Study the drawing (mm; zero at the part's minimum x, y, z) and answer. Coordinates: 2 decimals unless noted, no trailing zeros. Write each loop counter-clockwise with the first axis right and the second up, starting at its lowest first coordinate (ties: lowest second). Pieces come first, ordered by that corner, then holes. Notation, with made-up numbers: (-36, 87.25) -> (-21, 87.25) arc R28 ccw to (-21, 106.25) -> close; hole circle Ø1 at (-19.75, 72). An arc over 180 degrees is marked (long way). Answer in a Markdown table with one row per item. Add a question column.
Item 1: Given pin 1 Ø4 at (x, y) = (17, 5) entering from -Z; pin 2 Ø1 at (y, z) = (4.5, 19.5) entering from +X; pin 3 Ø6 at (x, z) = (146.05, 6.35) entering from +Y, each flat-ended and moving along its own axis, determine where each tip first touches the part or whether it passes through.
Item 2: Section D-D on x = 123 is taken. Write down the section's boundary in (y, z), then the cut area to 3 significant figures.
Item 3: Section C-C on z = 90.5 is taken. Write down the section's boundary in (x, y), then the cut area to 3 significant figures.
Item 4: Section A-A on x = 6.35 is taken. Write down the section's boundary in (y, z), then the cut area to 3 significant figures.
Item 5: Straight lines are drawn through the part: line 1 (Z direction, x = 6.35, y = 1.85); line 2 (Z direction, x = 82, y = 3). For each, find the intervals that lie inside material, in ascending order. Write a range as from..to.
Item 6: Section B-B on z = 6.35 is taken. Write down the section's boundary in (x, y).
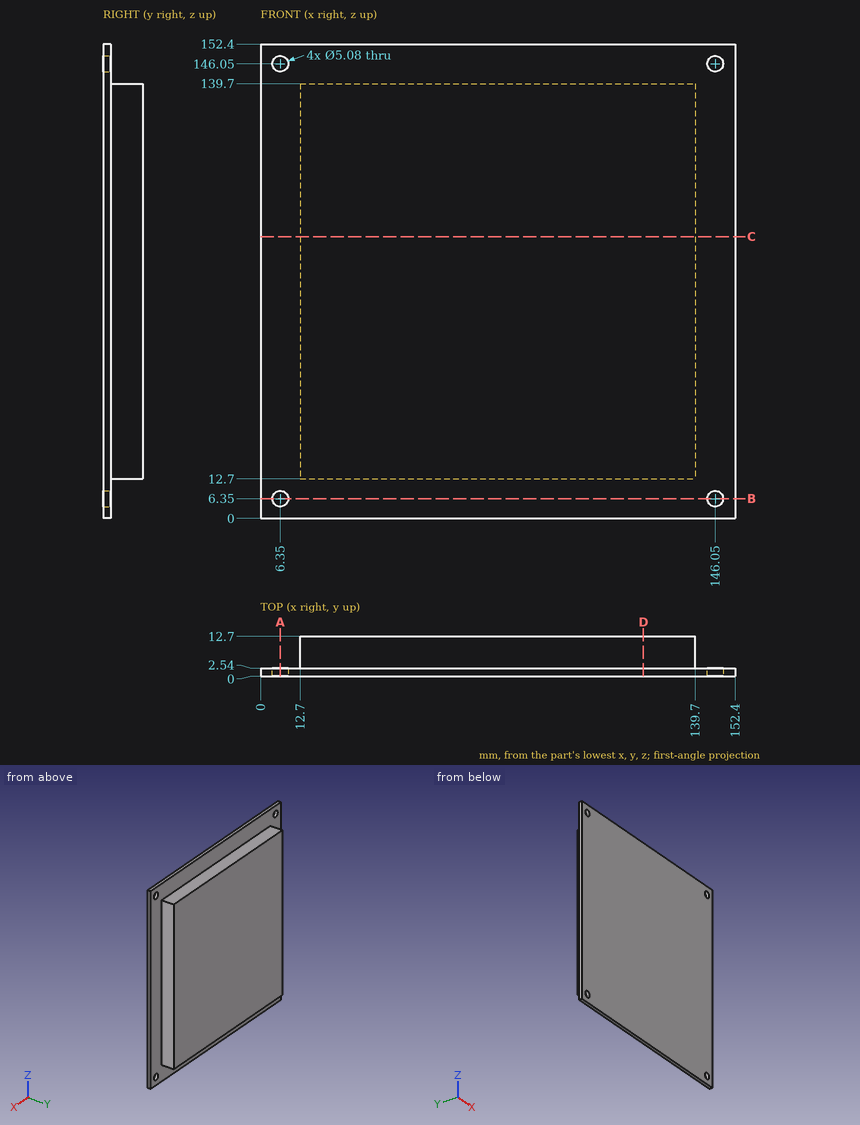
Results below:
| question | item | result |
|---|---|---|
| 1 | pin 1 | stops at z = 12.7 |
| 1 | pin 2 | stops at x = 139.7 |
| 1 | pin 3 | stops at y = 2.54 |
| 2 | outline | (0, 0) -> (2.54, 0) -> (2.54, 12.7) -> (12.7, 12.7) -> (12.7, 139.7) -> (2.54, 139.7) -> (2.54, 152.4) -> (0, 152.4) -> close |
| 2 | area | 1,680 mm2 |
| 3 | outline | (0, 0) -> (152.4, 0) -> (152.4, 2.54) -> (139.7, 2.54) -> (139.7, 12.7) -> (12.7, 12.7) -> (12.7, 2.54) -> (0, 2.54) -> close |
| 3 | area | 1,680 mm2 |
| 4 | outline | (0, 0) -> (2.54, 0) -> (2.54, 3.81) -> (0, 3.81) -> close; (0, 8.89) -> (2.54, 8.89) -> (2.54, 143.51) -> (0, 143.51) -> close; (0, 148.59) -> (2.54, 148.59) -> (2.54, 152.4) -> (0, 152.4) -> close |
| 4 | area | 361 mm2 |
| 5 | line 1 | z = 0..3.81, 8.89..143.51, 148.59..152.4 |
| 5 | line 2 | z = 12.7..139.7 |
| 6 | outline | (0, 0) -> (3.81, 0) -> (3.81, 2.54) -> (0, 2.54) -> close; (8.89, 0) -> (143.51, 0) -> (143.51, 2.54) -> (8.89, 2.54) -> close; (148.59, 0) -> (152.4, 0) -> (152.4, 2.54) -> (148.59, 2.54) -> close |
